The listing builds one solid part. Answer for the finished solid, in the listing's coordinates (mm). Face numbers are marked on the shaded views. Round coordinates to 2 decimals unless told otherwise and drop trailing zeros. Write each loop counter-clockwise with the first axis right and the second up, starting at its lowest first coordinate (ties: lowest second). Pieces come first, ordered by that corner, then holes.
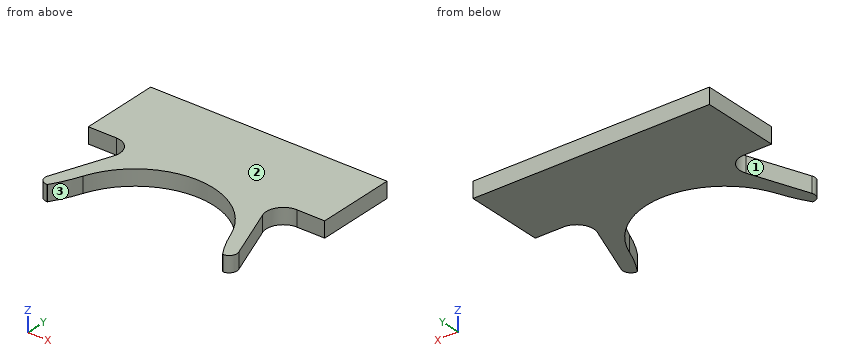
from build123d import *

# Parameters (mm, degrees)
EXTRUDE_1_DEPTH = 4


with BuildPart() as part:
    # 草图1 → 凸台-拉伸1 (new body)
    with BuildSketch(Plane.XY):
        with BuildLine():
            Line((-22.239358256, 0), (-22.36290973, 0))
            ThreePointArc((-22.36290973, 0), (-24.004989759, 0.858258708), (-24.237740304, 2.696426821))
            Line((-24.237740304, 2.696426821), (-18.862727252, 17.166344555))
            ThreePointArc((-18.862727252, 17.166344555), (-19.366277535, 21.143177652), (-22.918878713, 23))
            Line((-22.918878713, 23), (-30, 23))
            Line((-30, 23), (-30, 43))
            Line((-30, 43), (30, 43))
            Line((30, 43), (30, 23))
            Line((30, 23), (22.918878713, 23))
            ThreePointArc((22.918878713, 23), (19.366277535, 21.143177652), (18.862727252, 17.166344555))
            Line((18.862727252, 17.166344555), (24.237740304, 2.696426821))
            ThreePointArc((24.237740304, 2.696426821), (24.004989759, 0.858258708), (22.36290973, 0))
            Line((22.36290973, 0), (22.239358256, 0))
            ThreePointArc((22.239358256, 0), (20.299537687, 3.412102539), (18.731211271, 7.010115856))
            ThreePointArc((18.731211271, 7.010115856), (0, 20), (-18.731211271, 7.010115856))
            ThreePointArc((-18.731211271, 7.010115856), (-20.299537687, 3.412102539), (-22.239358256, 0))
        make_face()
    extrude(amount=EXTRUDE_1_DEPTH)


solid = part.part
1. Section C-C on y = 4 is taken. Determine the outline of the cut face in (x, z), plus the area to 3 significant figures.
Geometry says:
outline: (-23.75, 0) - (-20.01, 0) - (-20.01, 4) - (-23.75, 4) - close; (20.01, 0) - (23.75, 0) - (23.75, 4) - (20.01, 4) - close
area: 29.9 mm2
2. Section A-A on x = -21 is taken. Determine the outline of the cut face in (y, z).
Geometry says:
outline: (2.08, 0) - (11.41, 0) - (11.41, 4) - (2.08, 4) - close; (22.55, 0) - (43, 0) - (43, 4) - (22.55, 4) - close
3. For a pull along X with two mould halves and no side action, classify the marked faces 1, 2 and 3 as released by +X, released by -X, zero draft, split by the parting line, or undercut.
Geometry says:
face 1: released by -X
face 2: zero draft
face 3: undercut
4. Given pin 1 (1.2 mm diameter, centred on x = -25.5, z = 2, fed in from -Y), flat-ended and moving along its own axis, determine where the tip first touches the part or whether it passes through.
Geometry says:
pin 1: stops at y = 23
5. Section D-D on x = -11 is taken. Determine the outline of the cut face in (y, z), plus the area to 3 significant figures.
Geometry says:
outline: (16.7, 0) - (43, 0) - (43, 4) - (16.7, 4) - close
area: 105 mm2
6. Section B-B on z = 1.45 is taken. Determine the outline of the cut face in (x, y).
Geometry says:
outline: (-30, 23) - (-22.92, 23) arc R4.33 cw to (-18.86, 17.17) - (-24.24, 2.7) arc R2 ccw to (-22.36, 0) - (-22.24, 0) arc R37.08 ccw to (-18.73, 7.01) arc R20 cw to (18.73, 7.01) arc R37.08 ccw to (22.24, 0) - (22.36, 0) arc R2 ccw to (24.24, 2.7) - (18.86, 17.17) arc R4.33 cw to (22.92, 23) - (30, 23) - (30, 43) - (-30, 43) - close
7. Straight lines are drawn through the part: line 1 along X through (y, z) = (15, 2.3); line 2 along Y through (x, z) = (7, 1.7) (3 decimals); line 3 along Y through (x, z) = (-7.5, 3.15). For each, find the intervals that lie inside material, in ascending order.
Geometry says:
line 1: x = -19.67 to -13.23, 13.23 to 19.67
line 2: y = 18.735 to 43
line 3: y = 18.54 to 43
